Verification items for the finished model (mm, model axes). A direction names the side the tool comes from. Round coordinates to 2 decimals unless told otherwise and drop trailing zeros. Write each loop counter-clockwise with the first axis right and the second up, starting at its lowest first coordinate (ties: lowest second). Pieces come first, ordered by that corner, then holes. Notation, with made-up numbers: (88, 0.5) - (93, 0.5) arc R15 cw to (93, 24.5) - close; hole circle Ø10 at (-24.75, 5). An arc over 180 degrees is marked (long way). Answer as a JSON object with one key per item and string values.
```python
from build123d import *

# Parameters (mm, degrees)
F0_R     = 12.699304
F3_W     = 27.652487
F3_H     = 67.384638
F4_DEPTH = 25.4
F5_W     = 8.52412
F5_H     = 36.622613
F6_DEPTH = 11.176


with BuildPart() as f2:
    # F0 (on Front) → F2 (revolve)
    with BuildSketch(Plane.XZ):
        with Locations((0.033883, 0.343613)):
            Circle(F0_R)
    revolve(axis=Axis((-22.052867, 0, -26.479952), (-0.010936, 0, -0.99994)))

    # F3 (on Top) → F4 (join)
    with BuildSketch(Plane.XY):
        with Locations((-55.423274, -0.157852)):
            Rectangle(F3_W, F3_H)
    extrude(amount=F4_DEPTH)

    # F5 (on face) → F6 (join)
    with BuildSketch(Plane.XY.offset(25.4)):
        with Locations((-57.021674, -1.647932)):
            Rectangle(F5_W, F5_H)
    extrude(amount=F6_DEPTH)


solid = f2.part
```
1. Go/stop test with flat-tipped pins: pin 1 (2 mm diameter, centred on x = -7.5, y = 22, fed in from +Z); pin 2 (20.5 mm diameter, centred on x = -58, z = 11.5, fed in from +Y); pin 3 (20.5 mm diameter, centred on y = 12, z = 17, fed in from +X). Record where each tip stops, or that it passes through.
Completed:
{"pin 1": "stops at z = 12.68", "pin 2": "stops at y = 33.53", "pin 3": "stops at x = 9.49"}
2. Cross-section at A-A (z = 24). Record the boundary of the cut face in (x, y), plus the area to 3 significant figures.
Completed:
{"outline": "(-69.25, -33.85) - (-41.6, -33.85) - (-41.6, 33.53) - (-69.25, 33.53) - close", "area": "1,860 mm^2"}
3. Mould release check, pull along X, two halves, no side actions. Record for faces 1 (the face through (-41.597, -1, 15)), 2 (the face through (-61.284, -2, 31)), 3 (the face through (-57, -19.959, 31)): released by +X, released by -X, zero draft, split by the parting line, or undercut.
Completed:
{"face 1": "undercut", "face 2": "released by -X", "face 3": "zero draft"}
4. Material ranges on probe 1 along Y at (x, z) = (-57.5, 20.5); probe 2 along X at (y, z) = (-23.5, 14.5); probe 3 along Z at (x, y) = (-63, 11), recorded low to high. Write a range as from..to.
Completed:
{"probe 1": "y = -33.85..33.53", "probe 2": "x = -69.25..-41.6", "probe 3": "z = 0..25.4"}
5. Access from +Z, -Z, +X, -X, +Y, -Y to the whole of each face (thin tool, end or side, straight path). Record for faces 4 (the face through (-56, -33.85, 13)), 5 (the face through (-59, 0, 0)), 6 (the face through (-56, 33.534, 13)), 7 (the face through (-57, 16.663, 31)), 8 (the face through (-52.76, -2, 31)).
Completed:
{"face 4": "+Z, -Z, -X, -Y", "face 5": "-Z, -X", "face 6": "+Z, -Z, -X, +Y", "face 7": "+Z, +X, -X, +Y", "face 8": "+Z, +X, +Y, -Y"}
